Geometry: final body of the model. Coordinates: model frame, mm. Face numbers are marked on the shaded views. Give positions to 0.01 mm unless a question says otherwise; leave off trailing zeros. Order: outer loops, then holes, each group sorted by start corner. A loop starts at its lowest first (then second) coordinate and runs counter-clockwise, first axis right, second up. Notation, with made-up numbers: (-31, -11.5) -> (14, -11.5) arc R14 ccw to (14, 0.5) -> close; hole circle Ø5 at (54.25, 80.5). An arc over 180 degrees is marked (long way). Write item = value, one per line.
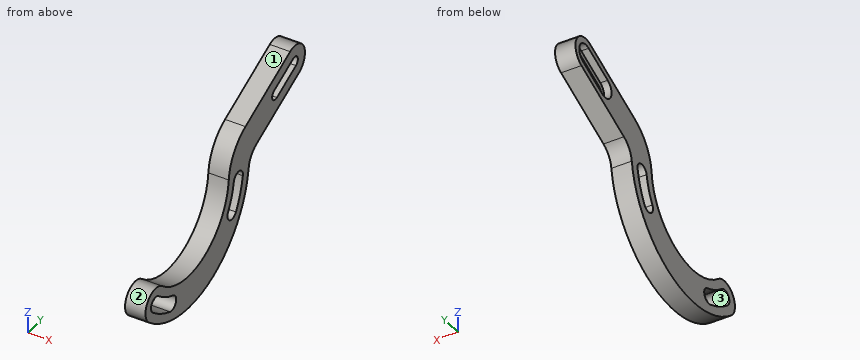
```python
from build123d import *

# Parameters (mm, degrees)
BOSS_EXTRUDE1_DEPTH = 9
FILLET1_R           = 10
CUT_EXTRUDE1_DEPTH  = 3.25


with BuildPart() as part:
    # Sketch2 → Boss-Extrude1 (new body)
    with BuildSketch(Plane(origin=(0, 0, 0), x_dir=(0, 0, -1), z_dir=(1, 0, 0))):
        with BuildLine():
            Line((-30.009207192, 73.421599264), (-14.966983891, 41.163447295))
            ThreePointArc((-14.966983891, 41.163447295), (-7.925043754, 32.797065521), (2.36792839, 29.103829905))
            ThreePointArc((2.36792839, 29.103829905), (26.999530596, 11.120492238), (22.178254162, -18.993815897))
            ThreePointArc((22.178254162, -18.993815897), (22.974363729, -29.286833411), (33.267381244, -28.490723845))
            ThreePointArc((33.267381244, -28.490723845), (39.862888041, 18.149108987), (0.354910699, 43.798562059))
            Line((0.354910699, 43.798562059), (-16.414590386, 79.76087319))
            ThreePointArc((-16.414590386, 79.76087319), (-26.381535752, 83.388544629), (-30.009207192, 73.421599264))
        make_face()
        with BuildLine():
            ThreePointArc((-14.612962522, 63.829641692), (-15.773817383, 60.640219175), (-18.9632399, 61.801074036))
            Line((-18.9632399, 61.801074036), (-25.387037478, 75.576952399))
            ThreePointArc((-25.387037478, 75.576952399), (-24.226182617, 78.766374916), (-21.0367601, 77.605520055))
            Line((-21.0367601, 77.605520055), (-14.612962522, 63.829641692))
        make_face(mode=Mode.SUBTRACT)
        with BuildLine():
            ThreePointArc((5.435407174, 32.75204343), (2.720199354, 36.547784002), (6.515939926, 39.262991823))
            ThreePointArc((6.515939926, 39.262991823), (13.612401704, 37.399766307), (20.246265091, 34.265562156))
            ThreePointArc((20.246265091, 34.265562156), (21.408669119, 29.745737284), (16.888844247, 28.583333256))
            ThreePointArc((16.888844247, 28.583333256), (11.355068758, 31.19779501), (5.435407174, 32.75204343))
        make_face(mode=Mode.SUBTRACT)
        with BuildLine():
            ThreePointArc((30.229264235, -25.888831256), (25.576256317, -26.248716403), (25.216371171, -21.595708485))
            ThreePointArc((25.216371171, -21.595708485), (28.752043406, -16.6), (31.310617746, -11.040163783))
            ThreePointArc((31.310617746, -11.040163783), (35.52018338, -9.025329503), (37.53501766, -13.234895137))
            ThreePointArc((37.53501766, -13.234895137), (34.467811071, -19.9), (30.229264235, -25.888831256))
        make_face(mode=Mode.SUBTRACT)
    extrude(amount=BOSS_EXTRUDE1_DEPTH)

    # Fillet1
    fillet1_edges = [part.edges().sort_by_distance(p)[0] for p in [
        (4.5, 43.798562059, -0.354910699),
    ]]
    fillet(fillet1_edges, radius=FILLET1_R)

    # Sketch3 → Cut-Extrude1 (cut)
    with BuildSketch(Plane.ZY):
        with BuildLine():
            Line((21.093063199, 60.80792112), (27.516860778, 74.583799483))
            ThreePointArc((27.516860778, 74.583799483), (25.219335532, 80.896198215), (18.906936801, 78.59867297))
            Line((18.906936801, 78.59867297), (12.483139222, 64.822794607))
            ThreePointArc((12.483139222, 64.822794607), (14.780664468, 58.510395875), (21.093063199, 60.80792112))
        make_face()
    extrude(amount=-CUT_EXTRUDE1_DEPTH, mode=Mode.SUBTRACT)


solid = part.part
```
1) Section query B-B (x = 5.75). Output: boundary loops of the cut face in (y, z).
Check sheet entries:
outline = (-28.49, -33.27) arc R43.8 ccw to (43.43, -5.65) arc R10 cw to (49.13, 2.13) -> (79.76, 16.41) arc R7.5 ccw to (73.42, 30.01) -> (41.16, 14.97) arc R21.01 ccw to (29.1, -2.37) arc R29.2 cw to (-18.99, -22.18) arc R7.3 ccw to start; hole (-25.89, -30.23) arc R39.8 ccw to (-13.23, -37.54) arc R3.3 ccw to (-11.04, -31.31) arc R33.2 cw to (-21.6, -25.22) arc R3.3 ccw to start; hole (28.58, -16.89) arc R3.3 ccw to (34.27, -20.25) arc R39.8 ccw to (39.26, -6.52) arc R3.3 ccw to (32.75, -5.44) arc R33.2 cw to start; hole (61.8, 18.96) arc R2.4 ccw to (63.83, 14.61) -> (77.61, 21.04) arc R2.4 ccw to (75.58, 25.39) -> close
2) Line query: line 1 (Y direction, x = 4.75, z = -25.5); line 2 (Z direction, x = 8.25, y = 73.5); line 3 (Y direction, x = 4.75, z = 16). Output: solid intervals per line, ascending. Write a range as from..to.
Check sheet entries:
line_1 = -30.7..-26.18, -21.26..-14.23, 14.23..35.61
line_2 = 13.5..19.12, 24.42..30.05
line_3 = 43.38..60.55, 66.8..78.87
3) Section query D-D (z = -36). Output: boundary loops of the cut face in (x, y), plus the area to 3 significant figures.
Check sheet entries:
outline = (0, -24.95) -> (9, -24.95) -> (9, -16.97) -> (0, -16.97) -> close; (0, -9.24) -> (9, -9.24) -> (9, 24.95) -> (0, 24.95) -> close
area = 379 mm²
4) Section query A-A (z = -12.5). Output: boundary loops of the cut face in (x, y).
Check sheet entries:
outline = (0, 26.39) -> (9, 26.39) -> (9, 30.76) -> (0, 30.76) -> close; (0, 37.79) -> (9, 37.79) -> (9, 41.98) -> (0, 41.98) -> close
5) Section query C-C (y = 67). Output: boundary loops of the cut face in (x, z), plus the area to 3 significant figures.
Check sheet entries:
outline = (0, 10.46) -> (9, 10.46) -> (9, 16.09) -> (3.25, 16.09) -> (3.25, 13.5) -> (0, 13.5) -> close; (0, 23.98) -> (3.25, 23.98) -> (3.25, 21.39) -> (9, 21.39) -> (9, 27.01) -> (0, 27.01) -> close
area = 84.4 mm²
6) First-contact query: P1, Ø5, axis at y = -6, z = -27.5, coming from the -X side; P2, Ø4, axis at x = 1, z = -32, coming from the +Y side; P3, Ø4, axis at x = 7.5, y = 55, coming from the +Z side; P4, Ø2, axis at x = 8, z = 13, coming from the -Y side. Flat tips, straight axial feed; report the tip coordinate or a pass-through.
Check sheet entries:
P1 = 0
P2 = 31.91
P3 = 22.35
P4 = 36.51
7) Mould query, pull axis Z, two halves, no side actions, for the marked faces 1, 2 and 3. Classes: +Z half, -Z half, draft (parallel to the pull), parting line (faces both ways), or undercut.
Check sheet entries:
face_1 = +Z half
face_2 = parting line
face_3 = undercut
